Drawing for the job (mm, zero at the part's lowest x, y, z). Round coordinates to 2 decimals unless told otherwise and drop trailing zeros. Write each loop counter-clockwise with the first axis right and the second up, starting at its lowest first coordinate (ties: lowest second). Pieces come first, ordered by that corner, then holes.
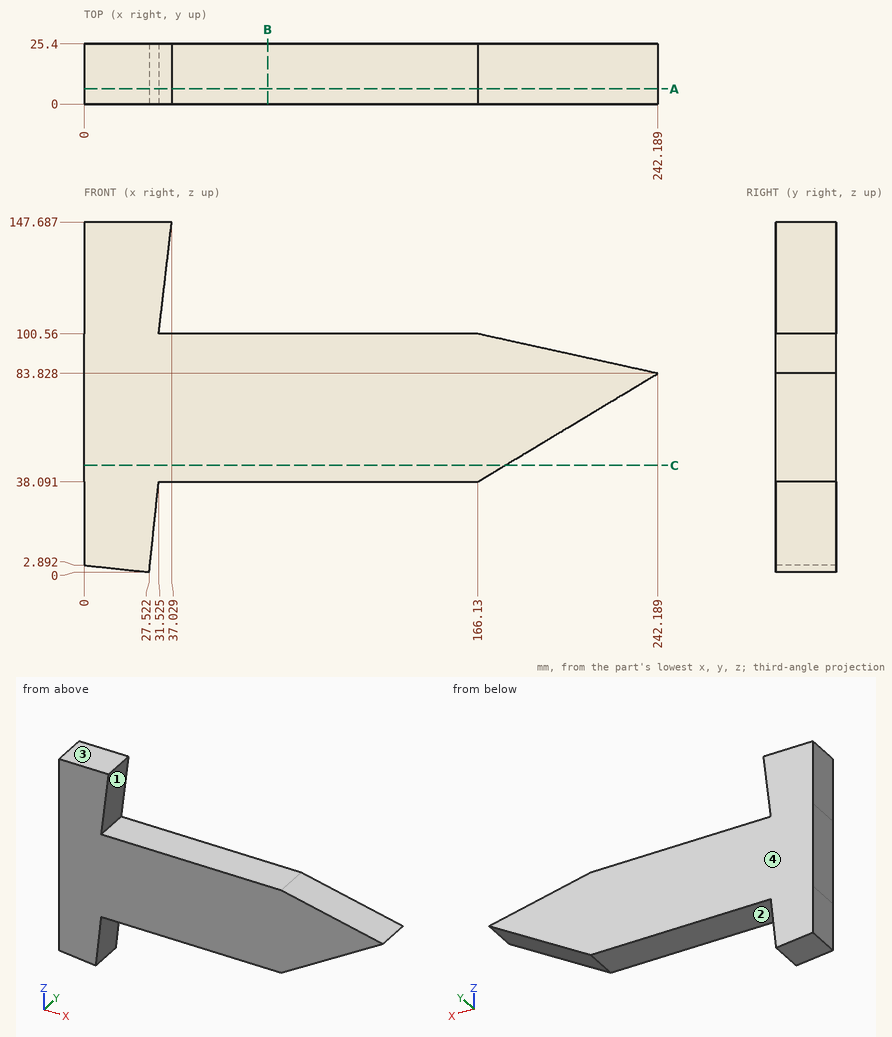
1) Cut at B-B on x = 77.5. List the corners of the cut face in (y, z), and give its area (3 significant figures).
2) Wall check: probe 1 along Z at (x, y) = (84.5, 12.5); probe 2 along Z at (x, y) = (12.5, 2); probe 3 along X at (y, z) = (14.5, 72). Give the ranges that are in metal, low to high.
3) Flat gauge pins, fed straight in: pin 1 Ø7.5 at (x, y) = (104, 9.5) entering from +Z; pin 2 Ø6 at (x, y) = (136, 22) entering from -Z; pin 3 Ø6 at (x, y) = (184, 7) entering from +Z. Where does each tip first touch, or does it go through?
4) Cut at A-A on y = 6.5. List the corners of the cut face in (x, z) (1 decimal).
5) Cut at C-C on z = 45. List the corners of the cut face in (x, y), and give its area (3 significant figures).
6) Pull direction Z, two halves, no side cores. Call the marked faces 1, 2, 3 and 4: released by +Z, released by -Z, zero draft, split by the parting line, or undercut.
Result sheet:
1. outline: (0, 38.09) - (25.4, 38.09) - (25.4, 100.56) - (0, 100.56) - close
1. area: 1,590 mm2
2. probe 1: z = 38.09 to 100.56
2. probe 2: z = 1.58 to 147.69
2. probe 3: x = 0 to 222.52
3. pin 1: stops at z = 100.56
3. pin 2: stops at z = 38.09
3. pin 3: stops at z = 97.29
4. outline: (0, 2.9) - (27.5, 0) - (31.5, 38.1) - (166.1, 38.1) - (242.2, 83.8) - (166.1, 100.6) - (31.5, 100.6) - (37, 147.7) - (0, 147.7) - close
5. outline: (0, 0) - (177.62, 0) - (177.62, 25.4) - (0, 25.4) - close
5. area: 4,510 mm2
6. face 1: undercut
6. face 2: released by -Z
6. face 3: released by +Z
6. face 4: zero draft
